The model under review builds one solid part; all positions refer to its coordinate system, in mm. Round coordinates to 2 decimals unless told otherwise and drop trailing zeros. One line per item, written item: value. Start each with the question number.
1) Mouldability with a two-part tool opening along X and no side actions: class faces 1 (the face through (-36, -1, 5.357)), 2 (the face through (-37, 0, 10)) as +X half, -X half, draft (parallel to the pull), parting line (faces both ways), or undercut.
2) For P1, Ø8, axis at x = -41.5, z = 7, coming from the +Y side; P2, Ø0.7, axis at x = -36, y = -2, coming from the +Z side; P3, Ø1.5, axis at y = -2, z = 13, coming from the -X side; P4, Ø1.5, axis at x = -52.5, y = -2, coming from the -Z side, all flat-tipped, find the tip position at first contact; note any pin that passes through.
3) Take a section at A-A, the plane z = 6. State how many separate pieces and enclosed holes the cut face has, and give its area (3 significant figures).
4) Wall thickness on probe 1 along X at (y, z) = (-1.2, 12.25); probe 2 along X at (y, z) = (-1.4, 11.75); probe 3 along X at (y, z) = (-2.65, 3.75): over which ranges is each line inside the solid? List them lowest first.
from build123d import *

# Parameters (mm, degrees)
F0_W        = 72.5492089987
F0_H        = 18.9791209996
F0_W_2      = 1.3700789067
F0_H_2      = 6.9912840748
F1_DEPTH    = 3
F2_T1_DEPTH = 82.5492089987
F2_T3_DEPTH = 28.9791209996
F3_R        = 0.5


# Not quite as in the source:
# - a fillet or chamfer that OpenCascade refuses, or shapes differently, is made with other operations: its cross-section is extruded or revolved along the edge and cut away or added


with BuildPart() as f1:
    # F0 (on Front) → F1 (new body)
    with BuildSketch(Plane.XZ):
        with Locations((-36.2746044993, 9.4895604998)):
            Rectangle(F0_W, F0_H)
        with BuildLine():
            Line((-40.2793404323, 5.3929338044), (-42.2747963845, 10.3801360367))
            Line((-42.2747963845, 10.3801360367), (-40.7738914752, 10.3801360367))
            Line((-40.7738914752, 10.3801360367), (-39.8264811924, 7.5537193204))
            add(Edge.make_bspline(
                [(-39.8264811924, 7.5537193204), (-39.70428108, 7.185681335), (-39.6597139803, 6.6825044018)],
                knots=[0, 0, 0, 1, 1, 1], degree=2))
            Line((-39.6597139803, 6.6825044018), (-39.632398661, 6.6825044018))
            add(Edge.make_bspline(
                [(-39.632398661, 6.6825044018), (-39.5835186161, 7.1454271804), (-39.439753778, 7.5537193204)],
                knots=[0, 0, 0, 1, 1, 1], degree=2))
            Line((-39.439753778, 7.5537193204), (-38.5095952758, 10.3801360367))
            Line((-38.5095952758, 10.3801360367), (-37.0403186308, 10.3801360367))
            Line((-37.0403186308, 10.3801360367), (-39.1651629373, 4.7143637688))
            add(Edge.make_bspline(
                [(-39.1651629373, 4.7143637688), (-39.458443207, 3.9279701046), (-39.9997178223, 3.5369297451)],
                knots=[0, 0, 0, 1, 1, 1], degree=2))
            add(Edge.make_bspline(
                [(-39.9997178223, 3.5369297451), (-40.5409924376, 3.1458893856), (-41.264129573, 3.1458893856)],
                knots=[0, 0, 0, 1, 1, 1], degree=2))
            add(Edge.make_bspline(
                [(-41.264129573, 3.1458893856), (-41.619228723, 3.1458893856), (-41.9599513892, 3.2235223981)],
                knots=[0, 0, 0, 1, 1, 1], degree=2))
            Line((-41.9599513892, 3.2235223981), (-41.9599513892, 4.3103845738))
            add(Edge.make_bspline(
                [(-41.9599513892, 4.3103845738), (-41.7126758677, 4.2514409902), (-41.4208332465, 4.2514409902)],
                knots=[0, 0, 0, 1, 1, 1], degree=2))
            add(Edge.make_bspline(
                [(-41.4208332465, 4.2514409902), (-41.0571082062, 4.2514409902), (-40.7853926623, 4.4742764892)],
                knots=[0, 0, 0, 1, 1, 1], degree=2))
            add(Edge.make_bspline(
                [(-40.7853926623, 4.4742764892), (-40.5136771183, 4.6971119882), (-40.36128639, 5.145658283)],
                knots=[0, 0, 0, 1, 1, 1], degree=2))
            Line((-40.36128639, 5.145658283), (-40.2793404323, 5.3929338044))
        make_face(mode=Mode.SUBTRACT)
        Polygon((-47.9362557073, 7.9533855702), (-47.9362557073, 5.3569925949), (-49.306334614, 5.3569925949), (-49.306334614, 11.9256080458), (-45.5411335052, 11.9256080458), (-45.5411335052, 10.7841152316), (-47.9362557073, 10.7841152316), (-47.9362557073, 9.0905654393), (-45.7079007174, 9.0905654393), (-45.7079007174, 7.9533855702), align=None, mode=Mode.SUBTRACT)
        with Locations((-43.6786600282, 8.8526346323)):
            Rectangle(F0_W_2, F0_H_2, mode=Mode.SUBTRACT)
        with BuildLine():
            Line((-31.6850784131, 8.6319556059), (-31.6850784131, 5.3569925949))
            Line((-31.6850784131, 5.3569925949), (-33.0551573198, 5.3569925949))
            Line((-33.0551573198, 5.3569925949), (-33.0551573198, 8.2912329397))
            add(Edge.make_bspline(
                [(-33.0551573198, 8.2912329397), (-33.0551573198, 8.8346640275), (-33.248521027, 9.1063795715)],
                knots=[0, 0, 0, 1, 1, 1], degree=2))
            add(Edge.make_bspline(
                [(-33.248521027, 9.1063795715), (-33.4418847342, 9.3780951154), (-33.8645533581, 9.3780951154)],
                knots=[0, 0, 0, 1, 1, 1], degree=2))
            add(Edge.make_bspline(
                [(-33.8645533581, 9.3780951154), (-34.4396127103, 9.3780951154), (-34.6955141221, 8.9942429978)],
                knots=[0, 0, 0, 1, 1, 1], degree=2))
            add(Edge.make_bspline(
                [(-34.6955141221, 8.9942429978), (-34.9514155338, 8.6103908802), (-34.9514155338, 7.7204865326)],
                knots=[0, 0, 0, 1, 1, 1], degree=2))
            Line((-34.9514155338, 7.7204865326), (-34.9514155338, 5.3569925949))
            Line((-34.9514155338, 5.3569925949), (-36.3214944405, 5.3569925949))
            Line((-36.3214944405, 5.3569925949), (-36.3214944405, 10.3801360367))
            Line((-36.3214944405, 10.3801360367), (-35.2748864195, 10.3801360367))
            Line((-35.2748864195, 10.3801360367), (-35.0908674267, 9.7375072106))
            Line((-35.0908674267, 9.7375072106), (-35.0146720626, 9.7375072106))
            add(Edge.make_bspline(
                [(-35.0146720626, 9.7375072106), (-34.7846483217, 10.1012322508), (-34.3828255993, 10.2874077161)],
                knots=[0, 0, 0, 1, 1, 1], degree=2))
            add(Edge.make_bspline(
                [(-34.3828255993, 10.2874077161), (-33.9810028769, 10.4735831814), (-33.4692000534, 10.4735831814)],
                knots=[0, 0, 0, 1, 1, 1], degree=2))
            add(Edge.make_bspline(
                [(-33.4692000534, 10.4735831814), (-32.5922345413, 10.4735831814), (-32.1386564772, 9.99987804)],
                knots=[0, 0, 0, 1, 1, 1], degree=2))
            add(Edge.make_bspline(
                [(-32.1386564772, 9.99987804), (-31.6850784131, 9.5261728986), (-31.6850784131, 8.6319556059)],
                knots=[0, 0, 0, 1, 1, 1], degree=2))
        make_face(mode=Mode.SUBTRACT)
        with BuildLine():
            Line((-25.6383293244, 8.6319556059), (-25.6383293244, 5.3569925949))
            Line((-25.6383293244, 5.3569925949), (-27.0084082311, 5.3569925949))
            Line((-27.0084082311, 5.3569925949), (-27.0084082311, 8.2912329397))
            add(Edge.make_bspline(
                [(-27.0084082311, 8.2912329397), (-27.0084082311, 8.8346640275), (-27.2017719383, 9.1063795715)],
                knots=[0, 0, 0, 1, 1, 1], degree=2))
            add(Edge.make_bspline(
                [(-27.2017719383, 9.1063795715), (-27.3951356454, 9.3780951154), (-27.8178042693, 9.3780951154)],
                knots=[0, 0, 0, 1, 1, 1], degree=2))
            add(Edge.make_bspline(
                [(-27.8178042693, 9.3780951154), (-28.3928636216, 9.3780951154), (-28.6487650333, 8.9942429978)],
                knots=[0, 0, 0, 1, 1, 1], degree=2))
            add(Edge.make_bspline(
                [(-28.6487650333, 8.9942429978), (-28.9046664451, 8.6103908802), (-28.9046664451, 7.7204865326)],
                knots=[0, 0, 0, 1, 1, 1], degree=2))
            Line((-28.9046664451, 7.7204865326), (-28.9046664451, 5.3569925949))
            Line((-28.9046664451, 5.3569925949), (-30.2747453518, 5.3569925949))
            Line((-30.2747453518, 5.3569925949), (-30.2747453518, 10.3801360367))
            Line((-30.2747453518, 10.3801360367), (-29.2281373307, 10.3801360367))
            Line((-29.2281373307, 10.3801360367), (-29.044118338, 9.7375072106))
            Line((-29.044118338, 9.7375072106), (-28.9679229738, 9.7375072106))
            add(Edge.make_bspline(
                [(-28.9679229738, 9.7375072106), (-28.7378992329, 10.1012322508), (-28.3360765105, 10.2874077161)],
                knots=[0, 0, 0, 1, 1, 1], degree=2))
            add(Edge.make_bspline(
                [(-28.3360765105, 10.2874077161), (-27.9342537882, 10.4735831814), (-27.4224509647, 10.4735831814)],
                knots=[0, 0, 0, 1, 1, 1], degree=2))
            add(Edge.make_bspline(
                [(-27.4224509647, 10.4735831814), (-26.5454854525, 10.4735831814), (-26.0919073884, 9.99987804)],
                knots=[0, 0, 0, 1, 1, 1], degree=2))
            add(Edge.make_bspline(
                [(-26.0919073884, 9.99987804), (-25.6383293244, 9.5261728986), (-25.6383293244, 8.6319556059)],
                knots=[0, 0, 0, 1, 1, 1], degree=2))
        make_face(mode=Mode.SUBTRACT)
    extrude(amount=F1_DEPTH)

    # F2: fillet of radius 2 on 4 edges, made by hand

    # F2_s2 → F2_t1 (cut)
    with BuildSketch(Plane.YZ.offset(-77.5492089987)):
        with BuildLine():
            add(Edge.make_bspline(
                [(-1, 18.9791209996), (-3, 18.9791209996), (-3, 16.9791209996)],
                knots=[0, 0, 0, 1, 1, 1], degree=2, weights=[1, 1, 1]))
            Line((-3, 16.9791209996), (-3, 18.9791209996))
            Line((-3, 18.9791209996), (-1, 18.9791209996))
        make_face()
        with BuildLine():
            add(Edge.make_bspline(
                [(-1, 0), (-3, 0), (-3, 2)],
                knots=[0, 0, 0, 1, 1, 1], degree=2, weights=[1, 1, 1]))
            Line((-3, 2), (-3, 0))
            Line((-3, 0), (-1, 0))
        make_face()
    extrude(amount=F2_T1_DEPTH, mode=Mode.SUBTRACT)

    # F2_s4 → F2_t3 (cut)
    with BuildSketch(Plane.XY.offset(-5)):
        with BuildLine():
            add(Edge.make_bspline(
                [(-72.5492089987, -1), (-72.5492089987, -3), (-70.5492089987, -3)],
                knots=[0, 0, 0, 1, 1, 1], degree=2, weights=[1, 1, 1]))
            Line((-70.5492089987, -3), (-72.5492089987, -3))
            Line((-72.5492089987, -3), (-72.5492089987, -1))
        make_face()
        with BuildLine():
            add(Edge.make_bspline(
                [(0, -1), (0, -3), (-2, -3)],
                knots=[0, 0, 0, 1, 1, 1], degree=2, weights=[1, 1, 1]))
            Line((-2, -3), (0, -3))
            Line((0, -3), (0, -1))
        make_face()
    extrude(amount=F2_T3_DEPTH, mode=Mode.SUBTRACT)

    # F3
    f3_edges = [f1.edges().sort_by_distance(p)[0] for p in [
        (-49.306335, -3, 8.6413),
        (-47.423734, -3, 11.925608),
        (-45.541134, -3, 11.354862),
        (-46.738695, -3, 10.784115),
        (-47.936256, -3, 9.93734),
        (-46.822078, -3, 9.090565),
        (-45.707901, -3, 8.521976),
        (-46.822078, -3, 7.953386),
        (-47.936256, -3, 6.655189),
        (-48.621295, -3, 5.356993),
    ]]
    fillet(f3_edges, radius=F3_R)


solid = f1.part
Checked values:
1. face 1: undercut
1. face 2: draft
2. P1: stops at y = 0
2. P2: stops at z = 18.92
2. P3: stops at x = -72.54
2. P4: stops at z = 0.01
3. separate pieces: 8
3. enclosed holes: 0
3. area: 186 mm2
4. probe 1: x = -72.54 to -44.36, -42.99 to -0.01
4. probe 2: x = -72.53 to -49.31, -45.54 to -44.36, -42.99 to -0.02
4. probe 3: x = -71.87 to -41.96, -39.75 to -0.68
